Geometry check sheet. Reference: the model listing, model coordinates, mm. Face numbers are marked on the shaded views. A direction names the side the tool comes from. Give positions to 0.01 mm unless a question says otherwise; leave off trailing zeros. Write each loop counter-clockwise with the first axis right and the second up, starting at its lowest first coordinate (ties: lowest second). Pieces come first, ordered by that corner, then holes. Notation, with made-up numbers: (32, -20.75) - (64, -20.75) arc R32 ccw to (64, 12.25) - close; hole circle Ø6 at (-32.75, 30). An arc over 180 degrees is marked (long way). Use a Markdown table: item, result.
Autodesk Inventor part; units mm, degrees
ref_plane "Work Plane1" through (12, 107, 55) normal (0, 1, 0) x (1, 0, 0)
ref_plane "YZ Plane" through (0, 0, 0) normal (1, 0, 0) x (0, 1, 0)
ref_plane "XZ Plane" through (0, 0, 0) normal (0, 1, 0) x (-1, 0, 0)
sketch "Sketch1" plane through (0, 0, 0) normal (0, 0, 1) x (1, 0, 0)
  line L0 (31, 0) -> (31, 12)
  line L1 (31, 12) -> (9, 12)
  line L2 (9, 12) -> (9, 82)
  line L3 (31, 0) -> (17, 0)
  line L4 (17, 0) -> (0, 0)
  line L5 (9, 82) -> (0, 82)
  line L6 (-31, 0) -> (-31, 12)
  line L7 (-31, 12) -> (-9, 12)
  line L8 (-9, 12) -> (-9, 82)
  line L9 (-31, 0) -> (-17, 0)
  line L10 (-17, 0) -> (0, 0)
  line L11 (-9, 82) -> (0, 82)
  point P0 (0, 0)
  dimension "d7" = 14
  dimension "d8" = 17
  dimension "d10" = 70
  dimension "d11" = 22
  dimension "d12" = 12
  dimension "d13" = 18
extrude "Extrusion1" add sketch "Sketch1" along normal mid plane 50
sketch "Sketch2" plane through (31, 0, 25) normal (1, 0, 0) x (0, 0, -1)
  line L0 (50, 82) -> (0, 82)
  circle A0 centre (25, -28) radius 28
  point P0 (25, 0)
  dimension "d17" = 56
extrude "Extrusion2" add sketch "Sketch2" along normal blind 3
sketch "Sketch3" plane through (31, 0, 25) normal (-1, 0, 0) x (0, 0, 1)
  arc A0 (-53, -28) -> (-25, 0) centre (-25, -28) ccw
  circle A1 centre (-25, -28) radius 28
  point P0 (-25, 0)
extrude "Extrusion3" add sketch "Sketch3" along normal blind 67
sketch "Sketch5" plane through (9, 12, 25) normal (1, 0, 0) x (0, 0, -1)
  line L0 (50, 70) -> (0, 70)
  circle A0 centre (25, 70) radius 25
  point P0 (25, -12)
  dimension "d24" = 50
extrude "Extrusion5" add sketch "Sketch5" along normal blind 3
sketch "Sketch6" plane through (9, 12, 25) normal (-1, 0, 0) x (0, 0, 1)
  arc A0 (0, 70) -> (-50, 70) centre (-25, 70) ccw
  circle A1 centre (-25, 70) radius 25
  point P0 (-25, -12)
  point P1 (0, 70)
extrude "Extrusion6" add sketch "Sketch6" along normal blind 43
sketch "Sketch7" plane through (-31, 12, 25) normal (0, 1, 0) x (1, 0, 0)
  point P0 (31, 25)
ref_plane "Work Plane1" through (12, 107, 55) normal (0, 1, 0) x (1, 0, 0)
sketch "Sketch10" plane through (12, 107, 55) normal (0, 1, 0) x (1, 0, 0)
  line L0 (-2.3312, -30.1107) -> (-2.219, -0.0002)
  line L1 (-2.219, -0.0002) -> (-14.1262, -0.0002)
  line L2 (-2.3312, -30.1107) -> (-14.238, -30.0664)
  line L3 (-44.0784, -29.9553) -> (-43.9668, 0.0445)
  line L4 (-43.9668, 0.0445) -> (-31.9669, -0.0002)
  line L5 (-44.0784, -29.9553) -> (-32.1716, -29.9996)
  line L6 (-14.1259, 55) -> (-31.9669, 55)
  line L7 (-2.219, 29.9997) -> (52.781, 29.9997) construction
  line L8 (-31.9669, -0.0002) -> (-31.9669, 55)
  line L9 (-14.1259, 55) -> (-14.1262, -0.0002)
  line L10 (-32.1716, -29.9996) -> (-14.238, -30.0664)
extrude "Extrusion8" add sketch "Sketch10" against normal blind 36
sketch "Sketch12" plane through (12, 82, 0) normal (1, 0, 0) x (0, 0, -1)
  circle A0 centre (0, 0) radius 12.5
  point P0 (0, -82)
  dimension "d48" = 25
sketch "Sketch13" plane through (34, -28, 0) normal (1, 0, 0) x (0, 0, -1)
  circle A0 centre (0, 0) radius 16
  point P0 (0, 28)
  dimension "d49" = 32
sketch "Sketch15" plane through (9.6688, 71, 85.1107) normal (1, 0, 0.0037) x (0.0037, 0, -1)
  line L0 (-0.0001, 36) -> (-0.0001, 0)
  circle A0 centre (-0.0001, 18) radius 18
  point P0 (85.0741, -71)
extrude "Extrusion9" add sketch "Sketch15" along normal blind 3
sketch "Sketch16" plane through (12.6688, 89, 85.1219) normal (1, 0, 0.0037) x (0.0037, 0, -1)
  circle A0 centre (0, 0) radius 18
  point P0 (85.0741, -89)
extrude "Extrusion10" add sketch "Sketch16" against normal blind 48
sketch "Sketch17" plane through (12, 107, 55) normal (0, 1, 0) x (1, 0, 0)
  line L0 (-32.1046, -11.9997) -> (-14.171, -12.0665)
  line L1 (-32.1046, -11.9997) -> (-32.1046, -64.3994)
  line L2 (-32.1046, -64.3994) -> (-14.171, -64.3994)
  line L3 (-14.171, -64.3994) -> (-14.171, -12.0665)
  line L4 (-14.171, -12.0665) -> (-32.1046, -11.9997)
  point P0 (-12, 55)
extrude "Extrusion11" cut sketch "Sketch17" against normal blind 48
sketch "Sketch18" plane through (12.6688, 89, 85.1219) normal (1, 0, 0.0037) x (0.0037, 0, -1)
  circle A0 centre (0, 0) radius 7.5
  point P0 (85.0741, -89)
  dimension "d56" = 15
extrude "Extrusion12" cut sketch "Sketch18" against normal blind 70
extrude "Extrusion13" cut sketch "Sketch12" against normal blind 70
extrude "Extrusion14" cut sketch "Sketch13" against normal blind 70
sketch "Sketch19" plane through (31, 0, 25) normal (1, 0, 0) x (0, 0, -1)
  line L0 (50, 12) -> (0, 12)
  line L1 (0, 12) -> (0, -21.7285)
  line L2 (0, -21.7285) -> (50, -21.7285)
  line L3 (50, -21.7285) -> (50, 12)
  line L4 (50, 12) -> (0, 12)
  point P0 (25, 0)
extrude "Extrusion15" add sketch "Sketch19" against normal blind 62
sketch "Sketch20" plane through (34, -28, 0) normal (1, 0, 0) x (0, 0, -1)
  circle A0 centre (0, 0) radius 16
  point P0 (0, 28)
extrude "Extrusion16" cut sketch "Sketch20" against normal blind 70
sketch "Sketch21" plane through (0, 0, 25) normal (0, 0, 1) x (1, 0, 0)
  line L0 (0, 0) -> (17, 0)
  line L1 (17, 0) -> (17, -69.3639)
  line L2 (17, -69.3639) -> (-1, -69.3639)
  line L3 (-1, -69.3639) -> (-18, -69.3639)
  line L4 (-18, -69.3639) -> (-18, 0)
  line L5 (-18, 0) -> (0, 0)
  dimension "d67" = 17
  dimension "d68" = 17
extrude "Extrusion17" cut sketch "Sketch21" along normal mid plane 150
properties part number "Sólido 2"
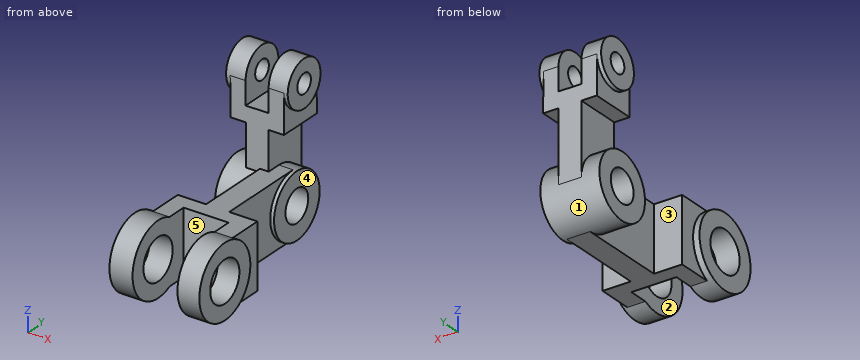
1) Section check B-B on z = -7. Count the separate pieces of the cut face and the enclosed holes in it, then the cut area to 3 significant figures.
Working result:
| item | result |
|---|---|
| separate pieces | 4 |
| enclosed holes | 0 |
| area | 3,740 mm² |
2) Mould release check, pull along X, two halves, no side actions. Record for the marked faces 4 and 5: pulls with the +X half, pulls with the -X half, needs draft (parallel to the pull), parting line crosses it, or undercut.
Working result:
| item | result |
|---|---|
| face 4 | pulls with the +X half |
| face 5 | undercut |
3) Material ranges on L1, parallel to Y at x = -10, z = 0; L2, parallel to X at y = -9, z = -18; L3, parallel to Y at x = 28.5, z = 0, recorded low to high. Write a range as from..to.
Working result:
| item | result |
|---|---|
| L1 | y = 0..12, 57..69.5, 94.5..107 |
| L2 | x = -36..-18, 17..34 |
| L3 | y = -56..-44, -12..12 |
4) Section check D-D on x = -6.5. Record the boundary of the cut face in (y, z), then the cut area to 3 significant figures.
Working result:
| item | result |
|---|---|
| outline | (0, -25) - (82, -25) arc R25 ccw to (107, 0) - (107, 67.05) - (71, 67.05) - (71, 25) - (0, 25) - close; hole circle Ø25 at (82, 0) |
| area | 6,240 mm² |
5) Set-up check for the marked faces 1, 2 and 3: record each of +Z, -Z, +X, -X, +Y, -Y from which the full face is reachable in a straight line by a thin tool's end or side.
Working result:
| item | result |
|---|---|
| face 1 | none |
| face 2 | +Z, -Z, -Y |
| face 3 | +Z, -Z, -X |
6) Depth check by flat-ended pin: P1, Ø10, axis at y = 90, z = 86.5, coming from the +X side; P2, Ø11, axis at y = 93.5, z = 86.5, coming from the +X side; P3, Ø10, axis at x = -19, z = 24.5, coming from the -Y side; P4, Ø2, axis at y = 9.5, z = -7, coming from the -X side. Enter the tip coordinate at first touch or a pass-through.
Working result:
| item | result |
|---|---|
| P1 | passes through |
| P2 | stops at x = 12.68 |
| P3 | stops at y = -48.09 |
| P4 | stops at x = -31 |
7) Section check A-A on x = -15.5. Record the boundary of the cut face in (y, z).
Working result:
| item | result |
|---|---|
| outline | (0, -25) - (12, -25) - (12, 25) - (0, 25) - close; (71, 22.45) arc R25 ccw (long way) to (107, 0) - (107, 67.02) - (71, 67.02) - close; hole circle Ø25 at (82, 0) |
